Read the model definition and answer for the solid it produces. Units are mm, in the model's axes. A direction names the side the tool comes from. Give positions to 0.01 mm unless a question says otherwise; leave off trailing zeros. Write each loop counter-clockwise with the first axis right and the second up, starting at its lowest first coordinate (ties: lowest second). Pieces come first, ordered by that corner, then holes. Notation, with made-up numbers: M -23.5,-39.75 L -16.5,-39.75 A11 ccw -16.5,-32.75 Z; hole C 88.25,20 d10. An arc over 180 degrees is marked long. Answer as CSV lines item,"result". Start each with the question number.
```python
from build123d import *

# Parameters (mm, degrees)
BOSS_EXTRUDE1_DEPTH = 50.8
BOSS_EXTRUDE2_DEPTH = 0.762
BOSS_EXTRUDE3_DEPTH = 0.762
SKETCH4_R           = 3.302
CUT_EXTRUDE1_DEPTH  = 82.319677815
SKETCH5_R           = 1.905
CUT_EXTRUDE2_DEPTH  = 81.845849887


with BuildPart() as part:
    # Sketch1 → Boss-Extrude1 (new body)
    with BuildSketch(Plane.XY):
        Polygon((0, 0), (38.1, 0), (38.1, 50.8), (37.338, 50.8), (37.338, 0.762), (0.762, 0.762), (0.762, 50.8), (0, 50.8), align=None)
    extrude(amount=BOSS_EXTRUDE1_DEPTH)

    # Sketch2 → Boss-Extrude2 (add)
    with BuildSketch(Plane.XY.offset(50.8)):
        Polygon((0.762, 0.762), (13.462, 0.762), (0.762, 13.462), align=None)
        Polygon((37.338, 0.762), (24.638, 0.762), (37.338, 13.462), align=None)
    extrude(amount=-BOSS_EXTRUDE2_DEPTH)

    # Sketch3 → Boss-Extrude3 (add)
    with BuildSketch(Plane(origin=(0, 0, 0), x_dir=(-1, 0, 0), z_dir=(0, 0, -1))):
        Polygon((-37.338, 13.462), (-37.338, 0.762), (-24.638, 0.762), align=None)
        Polygon((-0.762, 0.762), (-13.462, 0.762), (-0.762, 13.462), align=None)
    extrude(amount=-BOSS_EXTRUDE3_DEPTH)

    # Sketch4 → Cut-Extrude1 (cut, through all)
    with BuildSketch(Plane.ZY):
        with Locations((25.4, 36.624302666)):
            Circle(SKETCH4_R)
    extrude(amount=-CUT_EXTRUDE1_DEPTH, mode=Mode.SUBTRACT)

    # Sketch5 → Cut-Extrude2 (cut, through all)
    with BuildSketch(Plane(origin=(0, 0.762, 0), x_dir=(1, 0, 0), z_dir=(0, 1, 0))):
        with Locations(Location((9.525, -9.525, 0), (0, 0, 270))):
            Circle(SKETCH5_R)
        with Locations(Location((9.525, -41.275, 0), (0, 0, 270))):
            Circle(SKETCH5_R)
        with Locations(Location((28.575, -41.275, 0), (0, 0, 270))):
            Circle(SKETCH5_R)
        with Locations(Location((28.575, -9.525, 0), (0, 0, 270))):
            Circle(SKETCH5_R)
    extrude(amount=-CUT_EXTRUDE2_DEPTH, mode=Mode.SUBTRACT)


solid = part.part
```
1. Given pin 1 (12 mm diameter, centred on x = 10.5, z = 20, fed in from +Y), flat-ended and moving along its own axis, determine where the tip first touches the part or whether it passes through.
2. Find section B-B on y = 41. Determine the outline of the cut face in (x, z).
3. Find section A-A on z = 25.4. Determine the outline of the cut face in (x, y), then the cut area to 3 significant figures.
4. Find the intervals of material crossed by line 1 (X direction, y = 18.5, z = 31.5); line 2 (Z direction, x = 3, y = 6); line 3 (Y direction, x = 8.5, z = 13.5), in increasing order. Write a range as [from, to].
5. Find section D-D on x = 33. Determine the outline of the cut face in (y, z).
6. Determine the mould class of faces 4 (the face through (38.1, 25, 25)), 5 (the face through (29, 4.8, 0)), 6 (the face through (7.201, 7.023, 50.424)) for opening direction X: +X half, -X half, draft (parallel to the pull), parting line (faces both ways), or undercut.
7. Find section C-C on z = 37.5. Determine the outline of the cut face in (x, y), then the cut area to 3 significant figures.
8. For faces 1 (the face through (30.899, 7.023, 50.424)), 2 (the face through (19, 0, 25)), 3 (the face through (4, 4, 50.038)), determine the directions among +Z, -Z, +X, -X, +Y, -Y from which every point of the face is accessible in a straight line to the end or side of a thin tool.
Computed:
1,pin 1,"stops at y = 0.76"
2,outline,"M 0,0 L 0.76,0 L 0.76,50.8 L 0,50.8 Z; M 37.34,0 L 38.1,0 L 38.1,50.8 L 37.34,50.8 Z"
3,outline,"M 0,0 L 38.1,0 L 38.1,33.32 L 37.34,33.32 L 37.34,0.76 L 0.76,0.76 L 0.76,33.32 L 0,33.32 Z; M 0,39.93 L 0.76,39.93 L 0.76,50.8 L 0,50.8 Z; M 37.34,39.93 L 38.1,39.93 L 38.1,50.8 L 37.34,50.8 Z"
3,area,"95.2 mm^2"
4,line 1,"x = [0, 0.76], [37.34, 38.1]"
4,line 2,"z = [0, 0.76], [50.04, 50.8]"
4,line 3,"y = [0, 0.76]"
5,outline,"M 0,0 L 9.12,0 L 9.12,0.76 L 0.76,0.76 L 0.76,50.04 L 9.12,50.04 L 9.12,50.8 L 0,50.8 Z"
6,face 4,"+X half"
6,face 5,"draft"
6,face 6,"undercut"
7,outline,"M 0,0 L 38.1,0 L 38.1,50.8 L 37.34,50.8 L 37.34,0.76 L 0.76,0.76 L 0.76,50.8 L 0,50.8 Z"
7,area,"105 mm^2"
8,face 1,"+Z, -Z, +Y"
8,face 2,"+Z, -Z, +X, -X, -Y"
8,face 3,"+Y"
